CAD build for the part. Positions are in the model's coordinates, mm. Face numbers are marked on the shaded views. A direction names the side the tool comes from. Give positions to 0.01 mm unless a question says otherwise; leave off trailing zeros. Loops run counter-clockwise (first coordinate to the right, second up) from the corner with the lowest first, then second, coordinate; pieces in that order, holes last.
Item 1: Which spindle directions (+Z, -Z, +X, -X, +Y, -Y) get a long thin tool onto all of the face, cutting with end or side? Do the marked faces 5 and 6. Say none if no direction does.
Item 2: Probe probe 1 along Z at (x, y) = (-15.6, 40.85); probe 2 along Z at (x, y) = (-33, 42); probe 3 along Z at (x, y) = (18.5, 1.3). List the from-to ranges inside material, lowest first.
Item 3: Drop flat-ended pins along their axis: P1, Ø5, axis at x = -15.6, z = 22.75, coming from the -Y side; P2, Ø6, axis at y = 35.5, z = 37, coming from the -X side; P3, Ø12, axis at x = -17.5, y = 25.5, coming from the +Z side; P4, Ø6, axis at x = -18.5, z = 5, coming from the +Y side. Give the stop position or say it passes through.
Item 4: Saw through at A-A on x = -33.25. Give the cut face in (y, z), plus the area to 4 significant figures.
Item 5: Saw through at B-B on z = 38.25. Give the cut face in (x, y), plus the area to 4 significant figures.
Item 6: Saw through at C-C on y = 41.5. Give the number of separate pieces and of enclosed holes in the cut face, plus the area to 3 significant figures.
Item 7: Saw through at D-D on x = -0.1. Give the cut face in (y, z), plus the area to 3 significant figures.
Item 8: Mould opens along Z. For the marked faces 1, 2, 3 and 4 say: released by +Z, released by -Z, zero draft, split by the parting line, or undercut.
from build123d import *

# Parameters (mm, degrees)
SKETCH1_W           = 46.5
SKETCH1_H           = 19
SKETCH1_R           = 2.15
BOSS_EXTRUDE1_DEPTH = 5
BOSS_EXTRUDE2_DEPTH = 45
BOSS_EXTRUDE5_DEPTH = 5
CUT_EXTRUDE1_REACH  = 47
SKETCH7_R           = 11.5
SKETCH7_R_2         = 1.65
SKETCH8_W           = 24
SKETCH8_H           = 5
BOSS_EXTRUDE6_DEPTH = 20
CUT_EXTRUDE2_REACH  = 47
SKETCH9_R           = 2.5
CHAMFER1_SIZE       = 5
SKETCH10_R          = 3
CUT_EXTRUDE3_DEPTH  = 2
SKETCH12_R          = 3.75
CUT_EXTRUDE5_DEPTH  = 2
SKETCH13_R          = 3.75
CUT_EXTRUDE6_DEPTH  = 1


with BuildPart() as part:
    # Sketch1 → Boss-Extrude1 (new body)
    with BuildSketch(Plane(origin=(0, 0, 0), x_dir=(1, 0, 0), z_dir=(0, 1, 0))):
        Rectangle(SKETCH1_W, SKETCH1_H)
        with Locations((-18.5, 5)):
            Circle(SKETCH1_R, mode=Mode.SUBTRACT)
        with Locations((-18.5, -5)):
            Circle(SKETCH1_R, mode=Mode.SUBTRACT)
        with Locations((18.5, -5)):
            Circle(SKETCH1_R, mode=Mode.SUBTRACT)
        with Locations((18.5, 5)):
            Circle(SKETCH1_R, mode=Mode.SUBTRACT)
    extrude(amount=BOSS_EXTRUDE1_DEPTH)

    # Sketch2 → Boss-Extrude2 (add)
    with BuildSketch(Plane(origin=(0, 0, 0), x_dir=(1, 0, 0), z_dir=(0, 1, 0))):
        Polygon((28.25, 14.5), (28.25, -14), (-23.25, -14), (-23.25, -9.5), (23.25, -9.5), (23.25, 9.5), (-23.25, 9.5), (-23.25, 14.5), align=None)
    extrude(amount=BOSS_EXTRUDE2_DEPTH)

    # Sketch6 → Boss-Extrude5 (add)
    with BuildSketch(Plane(origin=(0, 45, 0), x_dir=(1, 0, 0), z_dir=(0, 1, 0))):
        Polygon((28.25, -14), (-23.25, -14), (-23.25, -9.5), (-43.25, -9.5), (-43.25, -59.5), (28.25, -59.5), align=None)
    extrude(amount=-BOSS_EXTRUDE5_DEPTH)

    # Sketch7 → Cut-Extrude1 (cut, up to next)
    with BuildSketch(Plane(origin=(0, 45, 0), x_dir=(1, 0, 0), z_dir=(0, 1, 0)), mode=Mode.PRIVATE) as cut_extrude1_sk1:
        with Locations((-0.1, -38.25)):
            Circle(SKETCH7_R)
    cut_extrude1_tool1 = extrude(cut_extrude1_sk1.sketch, amount=-CUT_EXTRUDE1_REACH, mode=Mode.PRIVATE) & part.part
    add(cut_extrude1_tool1.solids().sort_by_distance((-0.1, 45, 38.25))[0], mode=Mode.SUBTRACT)
    # Sketch7 → Cut-Extrude1 (cut, up to next)
    with BuildSketch(Plane(origin=(0, 45, 0), x_dir=(1, 0, 0), z_dir=(0, 1, 0)), mode=Mode.PRIVATE) as cut_extrude1_sk2:
        with Locations((-15.6, -22.75)):
            Circle(SKETCH7_R_2)
    cut_extrude1_tool2 = extrude(cut_extrude1_sk2.sketch, amount=-CUT_EXTRUDE1_REACH, mode=Mode.PRIVATE) & part.part
    add(cut_extrude1_tool2.solids().sort_by_distance((-15.6, 45, 22.75))[0], mode=Mode.SUBTRACT)
    # Sketch7 → Cut-Extrude1 (cut, up to next)
    with BuildSketch(Plane(origin=(0, 45, 0), x_dir=(1, 0, 0), z_dir=(0, 1, 0)), mode=Mode.PRIVATE) as cut_extrude1_sk3:
        with Locations((15.4, -22.75)):
            Circle(SKETCH7_R_2)
    cut_extrude1_tool3 = extrude(cut_extrude1_sk3.sketch, amount=-CUT_EXTRUDE1_REACH, mode=Mode.PRIVATE) & part.part
    add(cut_extrude1_tool3.solids().sort_by_distance((15.4, 45, 22.75))[0], mode=Mode.SUBTRACT)
    # Sketch7 → Cut-Extrude1 (cut, up to next)
    with BuildSketch(Plane(origin=(0, 45, 0), x_dir=(1, 0, 0), z_dir=(0, 1, 0)), mode=Mode.PRIVATE) as cut_extrude1_sk4:
        with Locations((15.4, -53.75)):
            Circle(SKETCH7_R_2)
    cut_extrude1_tool4 = extrude(cut_extrude1_sk4.sketch, amount=-CUT_EXTRUDE1_REACH, mode=Mode.PRIVATE) & part.part
    add(cut_extrude1_tool4.solids().sort_by_distance((15.4, 45, 53.75))[0], mode=Mode.SUBTRACT)
    # Sketch7 → Cut-Extrude1 (cut, up to next)
    with BuildSketch(Plane(origin=(0, 45, 0), x_dir=(1, 0, 0), z_dir=(0, 1, 0)), mode=Mode.PRIVATE) as cut_extrude1_sk5:
        with Locations((-15.6, -53.75)):
            Circle(SKETCH7_R_2)
    cut_extrude1_tool5 = extrude(cut_extrude1_sk5.sketch, amount=-CUT_EXTRUDE1_REACH, mode=Mode.PRIVATE) & part.part
    add(cut_extrude1_tool5.solids().sort_by_distance((-15.6, 45, 53.75))[0], mode=Mode.SUBTRACT)

    # Sketch8 → Boss-Extrude6 (add)
    with BuildSketch(Plane.ZY.offset(23.25)):
        with Locations((-2.5, 42.5)):
            Rectangle(SKETCH8_W, SKETCH8_H)
    extrude(amount=BOSS_EXTRUDE6_DEPTH)

    # Sketch9 → Cut-Extrude2 (cut, up to next)
    with BuildSketch(Plane(origin=(0, 45, 0), x_dir=(1, 0, 0), z_dir=(0, 1, 0)), mode=Mode.PRIVATE) as cut_extrude2_sk1:
        with Locations((-33.25, 2.5)):
            Circle(SKETCH9_R)
    cut_extrude2_tool1 = extrude(cut_extrude2_sk1.sketch, amount=-CUT_EXTRUDE2_REACH, mode=Mode.PRIVATE) & part.part
    add(cut_extrude2_tool1.solids().sort_by_distance((-33.25, 45, -2.5))[0], mode=Mode.SUBTRACT)
    # Sketch9 → Cut-Extrude2 (cut, up to next)
    with BuildSketch(Plane(origin=(0, 45, 0), x_dir=(1, 0, 0), z_dir=(0, 1, 0)), mode=Mode.PRIVATE) as cut_extrude2_sk2:
        with Locations((-33.25, -22.5)):
            Circle(SKETCH9_R)
    cut_extrude2_tool2 = extrude(cut_extrude2_sk2.sketch, amount=-CUT_EXTRUDE2_REACH, mode=Mode.PRIVATE) & part.part
    add(cut_extrude2_tool2.solids().sort_by_distance((-33.25, 45, 22.5))[0], mode=Mode.SUBTRACT)
    # Sketch9 → Cut-Extrude2 (cut, up to next)
    with BuildSketch(Plane(origin=(0, 45, 0), x_dir=(1, 0, 0), z_dir=(0, 1, 0)), mode=Mode.PRIVATE) as cut_extrude2_sk3:
        with Locations((-33.25, -47.5)):
            Circle(SKETCH9_R)
    cut_extrude2_tool3 = extrude(cut_extrude2_sk3.sketch, amount=-CUT_EXTRUDE2_REACH, mode=Mode.PRIVATE) & part.part
    add(cut_extrude2_tool3.solids().sort_by_distance((-33.25, 45, 47.5))[0], mode=Mode.SUBTRACT)

    # Chamfer1
    chamfer1_edges = [part.edges().sort_by_distance(p)[0] for p in [
        (28.25, 22.5, -14.5),
        (28.25, 20, 14),
        (-43.25, 42.5, 59.5),
        (28.25, 42.5, 59.5),
        (-43.25, 42.5, -14.5),
    ]]
    chamfer(chamfer1_edges, length=CHAMFER1_SIZE)

    # Sketch10 → Cut-Extrude3 (cut)
    with BuildSketch(Plane(origin=(0, 45, 0), x_dir=(1, 0, 0), z_dir=(0, 1, 0))):
        with Locations((-15.6, -22.75)):
            Circle(SKETCH10_R)
        with Locations((15.4, -22.75)):
            Circle(SKETCH10_R)
        with Locations((-15.6, -53.75)):
            Circle(SKETCH10_R)
        with Locations((15.4, -53.75)):
            Circle(SKETCH10_R)
    extrude(amount=-CUT_EXTRUDE3_DEPTH, mode=Mode.SUBTRACT)

    # Sketch12 → Cut-Extrude5 (cut)
    with BuildSketch(Plane.XZ):
        with Locations((-18.5, 5)):
            Circle(SKETCH12_R)
        with Locations((-18.5, -5)):
            Circle(SKETCH12_R)
        with Locations((18.5, -5)):
            Circle(SKETCH12_R)
        with Locations((18.5, 5)):
            Circle(SKETCH12_R)
    extrude(amount=-CUT_EXTRUDE5_DEPTH, mode=Mode.SUBTRACT)

    # Sketch13 → Cut-Extrude6 (cut)
    with BuildSketch(Plane(origin=(0, 45, 0), x_dir=(1, 0, 0), z_dir=(0, 1, 0))):
        with Locations((-33.25, 2.5)):
            Circle(SKETCH13_R)
        with Locations((-33.25, -22.5)):
            Circle(SKETCH13_R)
        with Locations((-33.25, -47.5)):
            Circle(SKETCH13_R)
    extrude(amount=-CUT_EXTRUDE6_DEPTH, mode=Mode.SUBTRACT)


solid = part.part
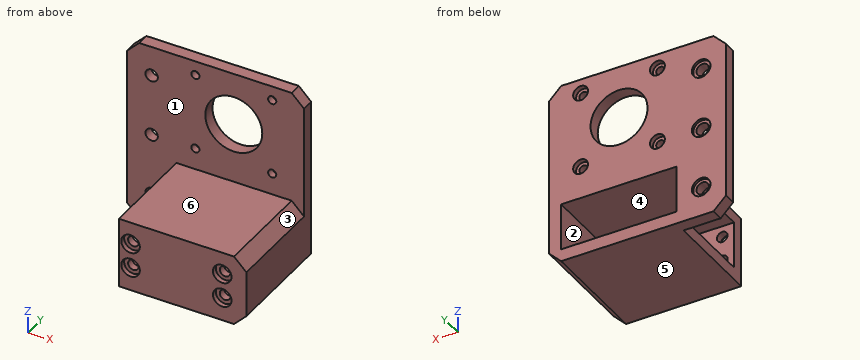
Results below:
1. face 5: -Z, +X, -X, +Y, -Y
1. face 6: +Z, +X, -X, -Y
2. probe 1: z = -14.5 to -9.5, 9.5 to 21.1, 24.4 to 52.1, 55.4 to 59.5
2. probe 2: z = -14.5 to -4.99, -0.01 to 20.01, 24.99 to 45.01, 49.99 to 59.5
2. probe 3: z = -14.5 to -8.75, -1.25 to 1.25, 8.75 to 14
3. P1: stops at y = 40
3. P2: passes through
3. P3: stops at z = 14
3. P4: stops at y = 5
4. outline: (40, -14.5) - (45, -14.5) - (45, -6.25) - (44, -6.25) - (44, -5) - (40, -5) - close; (40, 0) - (44, 0) - (44, 1.25) - (45, 1.25) - (45, 18.75) - (44, 18.75) - (44, 20) - (40, 20) - close; (40, 25) - (44, 25) - (44, 26.25) - (45, 26.25) - (45, 43.75) - (44, 43.75) - (44, 45) - (40, 45) - close; (40, 50) - (44, 50) - (44, 51.25) - (45, 51.25) - (45, 59.5) - (40, 59.5) - close
4. area: 287.5 mm2
5. outline: (-43.25, 40) - (-11.6, 40) - (-11.6, 45) - (-43.25, 45) - close; (11.4, 40) - (28.25, 40) - (28.25, 45) - (11.4, 45) - close
5. area: 242.5 mm2
6. separate pieces: 1
6. enclosed holes: 9
6. area: 3,850 mm2
7. outline: (0, -14.5) - (45, -14.5) - (45, -9.5) - (5, -9.5) - (5, 9.5) - (45, 9.5) - (45, 26.75) - (40, 26.75) - (40, 14) - (0, 14) - close; (40, 49.75) - (45, 49.75) - (45, 59.5) - (40, 59.5) - close
7. area: 635 mm2
8. face 1: zero draft
8. face 2: undercut
8. face 3: released by +Z
8. face 4: undercut
